Read the model definition and answer for the solid it produces. Units are mm, in the model's axes. A direction names the side the tool comes from. Give positions to 0.01 mm unless a question says otherwise; leave off trailing zeros. Use a Markdown table: item, result.
from build123d import *

# Parameters (mm, degrees)
F0_W             = 450
F0_H             = 450
F2_W             = 385
F2_H             = 385
F5_W             = 385
F5_H             = 385
F3_FACE_W        = 385
F3_FACE_H        = 385
F7_T             = 1
F12_COPIES_COUNT = 2
F12_COPIES_ANGLE = 90
F14_R            = 4.5
F15_DEPTH        = 420.4090421903
F16_R            = 4.5
F17_DEPTH        = 420.4090421903
F18_W            = 1
F18_H            = 5


# Not quite as in the source:
# - a feature of the source that left no trace in its solid (it failed there, or was rolled back) is left out
# - a pattern or mirror of a feature is missing from the dataset's text; its kind, count and spacing are read off the source's solid


with BuildPart() as f3:
    # F0 (on Front) → F3 section 0
    with BuildSketch(Plane.XZ):
        Rectangle(F0_W, F0_H)
    # F2 (on offset) → F3 section 1
    with BuildSketch(Plane.XZ.offset(-20)):
        Rectangle(F2_W, F2_H)
    loft()

    # F5 (on offset) → F6 section 0
    with BuildSketch(Plane.XZ.offset(-36)):
        Rectangle(F5_W, F5_H)
    # F3_face (on face) → F6 section 1
    with BuildSketch(Plane(origin=(0, 20, 0), x_dir=(-1, 0, 0), z_dir=(0, 1, 0))):
        Rectangle(F3_FACE_W, F3_FACE_H)
    loft()

    # F7
    f7_openings = [f3.faces().sort_by_distance(p)[0] for p in [
        (0, 0, 0),
        (0, 36, 0),
    ]]
    offset(amount=F7_T, openings=f7_openings, kind=Kind.INTERSECTION)

    # F8 (on face) → F10 (revolve, cut)
    with BuildSketch(Plane(origin=(-193.5, 0, 0), x_dir=(0, -1, 0), z_dir=(-1, 0, 0))):
        with BuildLine():
            Line((-20.558795194, -193.5), (-20.558795194, -192.5))
            add(Edge.make_bspline(
                [(-36, -192.5), (-20.558795194, -192.5)],
                knots=[0, 0, 0.9650753004, 0.9650753004], degree=1))
            Line((-36, -192.5), (-36, -193.5))
            Line((-36, -193.5), (-20.558795194, -193.5))
        make_face()
    revolve(axis=Axis((-193.5, 28.279397597, -193.5), (0, 1, 0)), mode=Mode.SUBTRACT)

    # F11 (on face) → F12 (revolve, cut)
    with BuildSketch(Plane.YZ.offset(193.5)):
        with BuildLine():
            Line((27.6298630059, -176.4289321881), (20.558795194, -183.5))
            Line((20.558795194, -183.5), (20.558795194, -192.5))
            add(Edge.make_bspline(
                [(36, -192.5), (20.558795194, -192.5)],
                knots=[0, 0, 0.9650753004, 0.9650753004], degree=1))
            Line((36, -192.5), (36, -170.9152411143))
            ThreePointArc((36, -170.9152411143), (33.0658481949, -175.5710584905), (27.6298630059, -176.4289321881))
        make_face()
        with BuildLine():
            add(Edge.make_bspline(
                [(36, -192.5), (20.558795194, -192.5)],
                knots=[0, 0, 0.9650753004, 0.9650753004], degree=1))
            Line((20.558795194, -192.5), (20.558795194, -193.5))
            Line((20.558795194, -193.5), (36, -193.5))
            Line((36, -193.5), (36, -192.5))
        make_face()
    f12 = revolve(axis=Axis((193.5, 28.279397597, -193.5), (0, 1, 0)), mode=Mode.SUBTRACT)

    # F12_copies: F12 ×2 about axis
    f12_copies_axis = Axis((1e-06, 0, -2.1e-05), (0, 1, 0))
    for i in range(1, F12_COPIES_COUNT):
        add(f12.rotate(f12_copies_axis, i * F12_COPIES_ANGLE / (F12_COPIES_COUNT - 1)), mode=Mode.SUBTRACT)

    # F12_copies1: F12 across plane
    add(f12.mirror(Plane(origin=(0, 0, 0), x_dir=(0.7071067823, 0, 0.7071067801), z_dir=(-0.7071067801, -6e-10, 0.7071067823))), mode=Mode.SUBTRACT)

    # F11 (on face) → F13 (revolve, cut)
    with BuildSketch(Plane.YZ.offset(193.5)):
        with BuildLine():
            Line((20.558795194, 193.5), (20.558795194, 192.5))
            add(Edge.make_bspline(
                [(36, 192.5), (20.558795194, 192.5)],
                knots=[0, 0, 0.9650753004, 0.9650753004], degree=1))
            Line((36, 192.5), (36, 193.5))
            Line((36, 193.5), (20.558795194, 193.5))
        make_face()
        with BuildLine():
            add(Edge.make_bspline(
                [(36, 192.5), (20.558795194, 192.5)],
                knots=[0, 0, 0.9650753004, 0.9650753004], degree=1))
            Line((20.558795194, 192.5), (20.558795194, 183.5))
            Line((20.558795194, 183.5), (27.6298630059, 176.4289321881))
            ThreePointArc((27.6298630059, 176.4289321881), (33.0658481949, 175.5710584905), (36, 170.9152411143))
            Line((36, 170.9152411143), (36, 192.5))
        make_face()
    revolve(axis=Axis((193.5, 28.279397597, 193.5), (0, 1, 0)), mode=Mode.SUBTRACT)

    # F14 (on face) → F15 (cut, through all)
    with BuildSketch(Plane(origin=(0, 0, -193.5), x_dir=(1, 0, 0), z_dir=(0, 0, -1))):
        with Locations((-25, -28)):
            Circle(F14_R)
        with Locations((25, -28)):
            Circle(F14_R)
        with Locations((-87.5, -28)):
            Circle(F14_R)
        with Locations((87.5, -28)):
            Circle(F14_R)
    extrude(amount=-F15_DEPTH, mode=Mode.SUBTRACT)

    # F16 (on face) → F17 (cut, through all)
    with BuildSketch(Plane(origin=(-193.5, 0, 0), x_dir=(0, -1, 0), z_dir=(-1, 0, 0))):
        with Locations((-28, 25)):
            Circle(F16_R)
        with Locations((-28, 87.5)):
            Circle(F16_R)
        with Locations((-28, -25)):
            Circle(F16_R)
        with Locations((-28, -87.5)):
            Circle(F16_R)
    extrude(amount=-F17_DEPTH, mode=Mode.SUBTRACT)

    # F19: sweep along a path in F19_path
    with BuildLine(Plane(origin=(-225, 0, 225), x_dir=(0, 0, -1), z_dir=(0, 1, 0))) as f19_path:
        Line((0, 0), (450, 0))
        Line((450, 0), (450, -450))
        Line((450, -450), (0, -450))
        Line((0, -450), (0, 0))
    # F18 (on Right) → F19 (sweep)
    with BuildSketch(Plane.YZ):
        with Locations((0.5, 227.5)):
            Rectangle(F18_W, F18_H)
    sweep(path=f19_path.line, transition=Transition.RIGHT)


solid = f3.part
Item 1: A tool of negligible diameter and unlimited length cuts with its end or side. For faces 1 (the face through (-193.5, 28, 3)), 2 (the face through (-193, 20.559, -191)), 3 (the face through (191, 20.559, -193)), from which of +Z, -Z, +X, -X, +Y, -Y can it reach the whole face along a straight path? Write none if from no direction.
Return value:
| item | result |
|---|---|
| face 1 | +Z, -Z, -X, +Y |
| face 2 | -Z, -X, +Y |
| face 3 | -Z, +X, +Y |
Item 2: Each of these flat-tipped pins is pushed along its axis until it touches: P1, Ø7.5, axis at y = 26, z = -57.5, coming from the -X side; P2, Ø11.5, axis at x = 87.5, y = 28, coming from the +Z side; P3, Ø7, axis at x = -25, y = 28, coming from the +Z side; P4, Ø17, axis at x = -36, y = 26.5, coming from the -Z side. Where does it stop, or does it pass through?
Return value:
| item | result |
|---|---|
| P1 | x = -193.5 |
| P2 | z = 193.5 |
| P3 | through |
| P4 | z = -197.66 |
Item 3: Straight lines are drawn through the part: line 1 along Z through (x, y) = (193.1, 28); line 2 along Z through (x, y) = (-174.5, 30). For each, find the intervals that lie inside material, in ascending order. Write a range as [from, to].
Return value:
| item | result |
|---|---|
| line 1 | [-176.52, -92], [-83, -29.5], [-20.5, 20.5], [29.5, 83], [92, 176.52] |
| line 2 | [-193.5, -192.5], [192.5, 193.5] |
Item 4: For a pull along X with two mould halves and no side action, classify faces 4 (the face through (-192.5, 28, 3)), 5 (the face through (3, 28, 193.5)), 6 (the face through (-209.169, 10.916, 3.154)), 7 (the face through (193.5, 28, -3)) as +X half, -X half, draft (parallel to the pull), parting line (faces both ways), or undercut.
Return value:
| item | result |
|---|---|
| face 4 | undercut |
| face 5 | draft |
| face 6 | -X half |
| face 7 | +X half |
